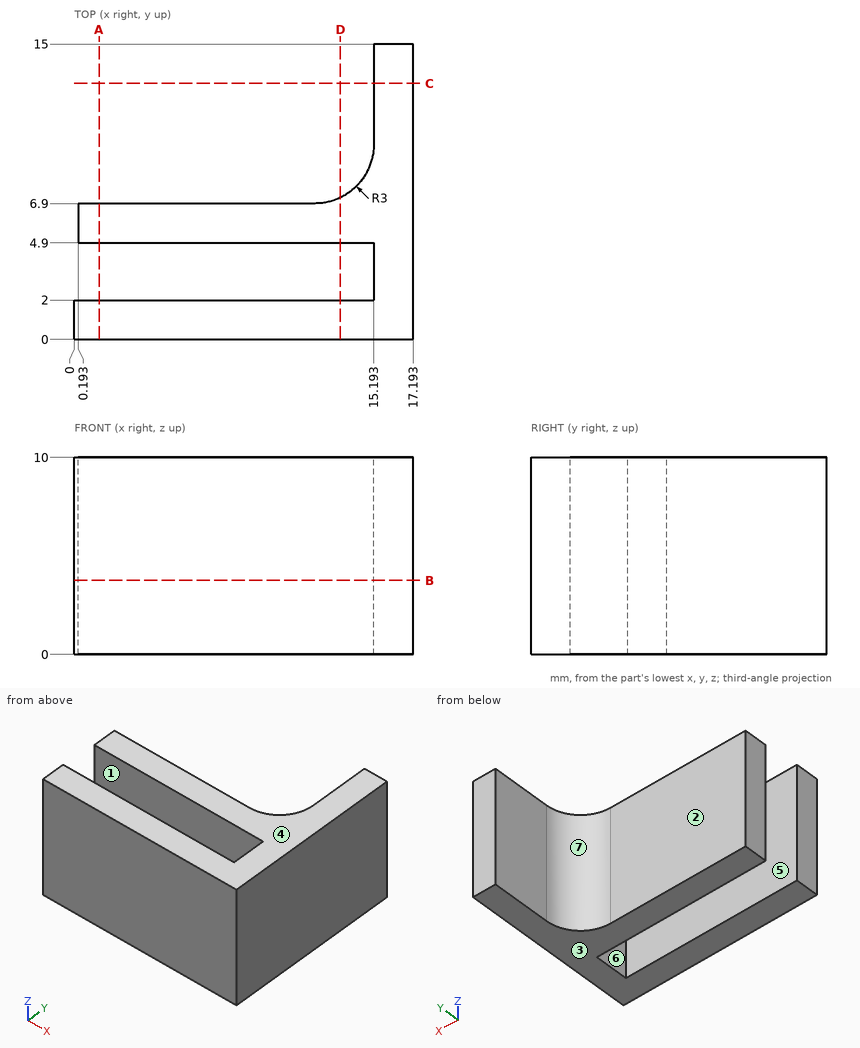
For this review, use the dimensioned drawing (mm, ordinates from the lowest corner) and the shaded views. A direction names the side the tool comes from. Round coordinates to 2 decimals unless told otherwise and drop trailing zeros. Order: outer loops, then holes, each group sorted by start corner. A loop starts at its lowest first (then second) coordinate and runs counter-clockwise, first axis right, second up.
1) For L1, parallel to Y at x = 2, z = 8.75; L2, parallel to X at y = 5, z = 4.75; L3, parallel to X at y = 13.25, z = 1.5, list the stretches that pass through material, from the lowest coordinate up.
The answers:
L1: y = 0 to 2, 4.9 to 6.9
L2: x = 0.19 to 17.19
L3: x = 15.19 to 17.19
2) Consider section A-A (x = 1.25). State the section outline as (y, z) points, plus the area to 3 significant figures.
The answers:
outline: (0, 0) - (2, 0) - (2, 10) - (0, 10) - close; (4.9, 0) - (6.9, 0) - (6.9, 10) - (4.9, 10) - close
area: 40.0 mm2
3) Consider section C-C (y = 13). State the section outline as (x, z) points.
The answers:
outline: (15.19, 0) - (17.19, 0) - (17.19, 10) - (15.19, 10) - close
4) Clearance check with flat-ended pins moving along their axes: pin 1 Ø0.6 at (y, z) = (6, 4) entering from -X; pin 2 Ø3 at (x, z) = (5.5, 5) entering from +Y; pin 3 Ø1.5 at (x, z) = (12.5, 4.5) entering from +Y. State where each tip first meets the part, or that it passes through.
The answers:
pin 1: stops at x = 0.19
pin 2: stops at y = 6.9
pin 3: stops at y = 7.09
5) Consider section D-D (x = 13.5). State the section outline as (y, z) points.
The answers:
outline: (0, 0) - (2, 0) - (2, 10) - (0, 10) - close; (4.9, 0) - (7.2, 0) - (7.2, 10) - (4.9, 10) - close
6) Draft analysis for pull direction Y (two halves, no side actions). For the marked faces 4, 5, 6 and 7, state which applies: released by +Y, released by -Y, zero draft, split by the parting line, or undercut.
The answers:
face 4: zero draft
face 5: undercut
face 6: undercut
face 7: released by +Y
7) Machinability: for the marked faces 1, 2 and 3, which of the approach directions +Z, -Z, +X, -X, +Y, -Y give a long, thin tool a straight path to every point of the face, cutting with its end or side? Answer none if there is none.
The answers:
face 1: +Z, -Z, -X
face 2: +Z, -Z, -X, +Y
face 3: -Z, +X, -X, +Y, -Y
8) Consider section B-B (z = 3.75). State the section outline as (x, y) points.
The answers:
outline: (0, 0) - (17.19, 0) - (17.19, 15) - (15.19, 15) - (15.19, 9.9) arc R3 cw to (12.19, 6.9) - (0.19, 6.9) - (0.19, 4.9) - (15.19, 4.9) - (15.19, 2) - (0, 2) - close
